Part model, mm, in its own coordinate system. A direction names the side the tool comes from. Give positions to 0.01 mm unless a question says otherwise; leave off trailing zeros. Order: outer loops, then holes, each group sorted by start corner. A loop starts at its lowest first (then second) coordinate and runs counter-clockwise, first axis right, second up. Notation, with made-up numbers: (46.5, -13) - (79.5, -13) arc R18 cw to (79.5, 1) - close; hole circle Ø5 at (9, 85.25). An arc over 180 degrees is marked (long way). Use a Markdown table: item, result. Add a question column.
from build123d import *

# Parameters (mm, degrees)
BARRER1_PROFILE_R            = 16
CROQUIS13_R                  = 12.462499683
SALIENTE_EXTRUIR1_DEPTH      = 30
SALIENTE_EXTRUIR2_DEPTH      = 2
SALIENTE_EXTRUIR2_DEPTH_BACK = 2
CROQUIS15_W                  = 22
CROQUIS15_H                  = 30
CROQUIS15_R                  = 5.5
REDONDEO1_R                  = 5


with BuildPart() as part:
    # Barrer1: sweep along a curve in space
    with BuildLine() as barrer1_path:
        Line((1505.090032208, -551.240046142, 2179.521039666), (1505.090032208, -605.839285822, 2179.521039666))
        ThreePointArc((1505.090032208, -605.839285822, 2179.521039666), (1505.090032208, -643.580384492, 2184.704091655), (1505.090032208, -678.526996356, 2199.869475793))
        Line((1505.090032208, -678.526996356, 2199.869475793), (1505.090032208, -717.466920568, 2223.52527976))
        ThreePointArc((1505.090032208, -717.466920568, 2223.52527976), (1505.090032208, -752.413532431, 2238.690663898), (1505.090032208, -790.154631102, 2243.873715887))
        Line((1505.090032208, -790.154631102, 2243.873715887), (1505.090032208, -1677.615278398, 2243.873715887))
        ThreePointArc((1505.090032208, -1677.615278398, 2243.873715887), (1505.090032208, -1712.970617457, 2229.229054946), (1505.090032208, -1727.615278398, 2193.873715887))
        Line((1505.090032208, -1727.615278398, 2193.873715887), (1505.090032208, -1727.615278398, 2163.873715887))
    # Barrer1 profile (on start of the path) → Barrer1 (sweep)
    with BuildSketch(Plane(origin=(1505.090032208, -551.240046142, 2179.521039666), x_dir=(0, 0, -1), z_dir=(0, -1, 0))):
        Circle(BARRER1_PROFILE_R)
    sweep(path=barrer1_path.line)

    # Croquis13 → Saliente-Extruir1 (add)
    with BuildSketch(Plane(origin=(0, -551.240046142, 0), x_dir=(1, 0, 0), z_dir=(0, 1, 0))):
        with Locations(Location((1505.090032208, -2179.521039666, 0), (0, 0, 270))):
            Circle(CROQUIS13_R)
    extrude(amount=SALIENTE_EXTRUIR1_DEPTH)

    # Croquis15 → Saliente-Extruir2 (add, two sides: drawn at the far end of the back side and taken through both)
    with BuildSketch(Plane.XY.offset(2179.521039666).offset(-SALIENTE_EXTRUIR2_DEPTH_BACK)):
        with Locations((1505.090032208, -506.240046142)):
            Rectangle(CROQUIS15_W, CROQUIS15_H)
        with Locations((1505.090032208, -499.005171033)):
            Circle(CROQUIS15_R, mode=Mode.SUBTRACT)
    extrude(amount=SALIENTE_EXTRUIR2_DEPTH + SALIENTE_EXTRUIR2_DEPTH_BACK)

    # Redondeo1
    # the kernel refuses this fillet: 5 mm, written as the material it takes off along each edge
    with BuildSketch(Plane(origin=(1505.090032208, -521.240046142, 2179.521039666), x_dir=(0, 0, 1), z_dir=(-1, 0, 0))) as redondeo1_piece_1_section:
        with BuildLine():
            CenterArc((12.462499683 - REDONDEO1_R, -REDONDEO1_R), REDONDEO1_R, 0, 90)
            Line((12.462499683 - REDONDEO1_R, 0), (12.462499683, 0))
            Line((12.462499683, 0), (12.462499683, -REDONDEO1_R))
        make_face()
    redondeo1_piece_1 = revolve(axis=Axis((1505.090032208, -521.240046142, 2179.521039666), (0, 1, 0)), mode=Mode.PRIVATE)
    redondeo1_piece_1 = split(redondeo1_piece_1, bisect_by=Plane(origin=(1512.161144528, -522.66682116, 2181.521039666), z_dir=(0, 0, 1)), keep=Keep.TOP, mode=Mode.PRIVATE)
    add(redondeo1_piece_1, mode=Mode.SUBTRACT)
    with BuildSketch(Plane(origin=(1505.090032208, -521.240046142, 2179.521039666), x_dir=(0, 0, 1), z_dir=(-1, 0, 0))) as redondeo1_piece_2_section:
        with BuildLine():
            CenterArc((12.462499683 - REDONDEO1_R, -REDONDEO1_R), REDONDEO1_R, 0, 90)
            Line((12.462499683 - REDONDEO1_R, 0), (12.462499683, 0))
            Line((12.462499683, 0), (12.462499683, -REDONDEO1_R))
        make_face()
    redondeo1_piece_2 = revolve(axis=Axis((1505.090032208, -521.240046142, 2179.521039666), (0, 1, 0)), mode=Mode.PRIVATE)
    redondeo1_piece_2 = split(redondeo1_piece_2, bisect_by=Plane(origin=(1505.090032208, -522.66682116, 2177.521039666), z_dir=(0, 0, -1)), keep=Keep.TOP, mode=Mode.PRIVATE)
    add(redondeo1_piece_2, mode=Mode.SUBTRACT)
    with BuildSketch(Plane(origin=(1505.090032208, -521.240046142, 2179.521039666), x_dir=(0, 0, 1), z_dir=(-1, 0, 0))) as redondeo1_piece_3_section:
        with BuildLine():
            CenterArc((12.462499683 - REDONDEO1_R, -REDONDEO1_R), REDONDEO1_R, 0, 90)
            Line((12.462499683 - REDONDEO1_R, 0), (12.462499683, 0))
            Line((12.462499683, 0), (12.462499683, -REDONDEO1_R))
        make_face()
    redondeo1_piece_3 = revolve(axis=Axis((1505.090032208, -521.240046142, 2179.521039666), (0, 1, 0)), mode=Mode.PRIVATE)
    redondeo1_piece_3 = split(redondeo1_piece_3, bisect_by=Plane(origin=(1516.090032208, -522.670135024, 2179.521039666), z_dir=(1, 0, 0)), keep=Keep.TOP, mode=Mode.PRIVATE)
    add(redondeo1_piece_3, mode=Mode.SUBTRACT)
    with BuildSketch(Plane(origin=(1505.090032208, -521.240046142, 2179.521039666), x_dir=(0, 0, 1), z_dir=(-1, 0, 0))) as redondeo1_piece_4_section:
        with BuildLine():
            CenterArc((12.462499683 - REDONDEO1_R, -REDONDEO1_R), REDONDEO1_R, 0, 90)
            Line((12.462499683 - REDONDEO1_R, 0), (12.462499683, 0))
            Line((12.462499683, 0), (12.462499683, -REDONDEO1_R))
        make_face()
    redondeo1_piece_4 = revolve(axis=Axis((1505.090032208, -521.240046142, 2179.521039666), (0, 1, 0)), mode=Mode.PRIVATE)
    redondeo1_piece_4 = split(redondeo1_piece_4, bisect_by=Plane(origin=(1494.090032208, -522.670134816, 2179.521039666), z_dir=(-1, 0, 0)), keep=Keep.TOP, mode=Mode.PRIVATE)
    add(redondeo1_piece_4, mode=Mode.SUBTRACT)


solid = part.part
1. Tool access for faces 1 (the face through (1509.9, -578.92, 2164.26)), 2 (the face through (1505.8, -1743.6, 2178.7)), 3 (the face through (1509.896, -1240.097, 2228.613)): list every direction of +Z, -Z, +X, -X, +Y, -Y with a clear straight run to the whole face (end or side of a thin tool).
2. Pin check, flat tips, straight feed: P1, Ø3, axis at y = -509, z = 2179.5, coming from the +X side; P2, Ø6, axis at x = 1496, z = 2227.5, coming from the -Y side; P3, Ø17.5, axis at x = 1507.5, y = -506.5, coming from the +Z side. Stop position of each tip, or through.
3. Mould opens along Y. For faces 4 (the face through (1505, -507, 2177.521)), 5 (the face through (1492, -551.24, 2180)), 6 (the face through (1515.904, -692.147, 2221.942)) say: released by +Y, released by -Y, zero draft, split by the parting line, or undercut.
4. Drill centre lines: probe 1 along Y at (x, z) = (1493, 2211); probe 2 along Y at (x, z) = (1509.5, 2190); probe 3 along X at (y, z) = (-1215, 2242). Where is each one in solid material? Low to high. Write a range as [from, to].
5. Cut at A-A (y = -1255). Write the cut outline in (x, z), plus the area to 3 significant figures.
Responses:
| question | item | result |
|---|---|---|
| 1 | face 1 | +Y |
| 1 | face 2 | -Z |
| 1 | face 3 | none |
| 2 | P1 | stops at x = 1516.09 |
| 2 | P2 | stops at y = -1733.79 |
| 2 | P3 | stops at z = 2181.52 |
| 3 | face 4 | zero draft |
| 3 | face 5 | released by +Y |
| 3 | face 6 | undercut |
| 4 | probe 1 | y = [-1735.62, -1713.23], [-717.03, -676.66] |
| 4 | probe 2 | y = [-1743, -1712.24], [-691.9, -523.12] |
| 4 | probe 3 | x = [1489.2, 1520.98] |
| 5 | outline | circle Ø32 at (1505.09, 2243.87) |
| 5 | area | 804 mm² |
